Design review of the part built by this model. Coordinates are the model's own, in mm. Coordinates: 2 decimals unless noted, no trailing zeros. Write each loop counter-clockwise with the first axis right and the second up, starting at its lowest first coordinate (ties: lowest second). Pieces come first, ordered by that corner, then holes.
Q1. For L1, parallel to Z at x = -53.73, y = 1.65 (3 decimals); L2, parallel to X at y = 0.75, z = -48.73 (3 decimals); L3, parallel to X at y = 1.7, z = -49, list the stretches that pass through material, from the lowest coordinate up.
Q2. For pin 1 Ø8 at (x, z) = (-26.5, -44) entering from -Y; pin 2 Ø1 at (x, y) = (-42, 1) entering from +Z; pin 3 Ø1 at (y, z) = (1, -48) entering from -X, all flat-tipped, find the tip position at first contact; note any pin that passes through.
Q3. Take a section at A-A, the plane y = 0.75. State how many separate pieces and enclosed holes the cut face has, plus the area to 3 significant figures.
Q4. Take a section at C-C, the plane x = -31.5. Write out the cut boundary in (y, z), plus the area to 3 significant figures.
Q5. Take a section at B-B, the plane z = -7. Write out the cut boundary in (x, y), plus the area to 3 significant figures.
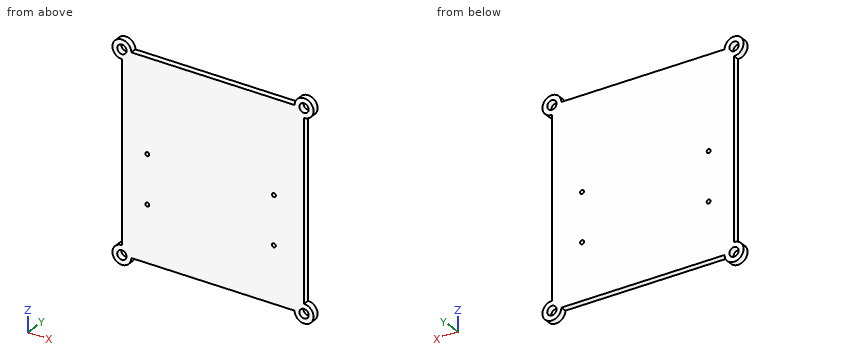
Autodesk Inventor part; units mm, degrees
ref_plane "YZ Plane" through (0, 0, 0) normal (1, 0, 0) x (0, 1, 0)
ref_plane "XZ Plane" through (0, 0, 0) normal (0, 1, 0) x (-1, 0, 0)
ref_plane "XY Plane" through (0, 0, 0) normal (0, 0, 1) x (1, 0, 0)
sketch "Sketch1" plane through (0, 0, 0) normal (0, 1, 0) x (-1, 0, 0)
  line L0 (0, 0) -> (65, 0)
  line L1 (65, 0) -> (65, -70)
  line L2 (65, -70) -> (0, -70)
  line L3 (0, -70) -> (0, 0)
  dimension "d0" = 65
  dimension "d1" = 70
extrude "Extrusion1" add sketch "Sketch1" along normal blind 2
sketch "Sketch2" plane through (0, 2, 0) normal (0, 1, 0) x (1, 0, 0)
  line L0 (0, 70) -> (-65, 70)
  line L1 (-32.5, 69) -> (-10.5, 69)
  line L2 (-32.5, 69) -> (-54.5, 69)
  line L3 (-10.5, 69) -> (-10.5, 55)
  line L4 (-10.5, 55) -> (-54.5, 55)
  line L5 (-54.5, 55) -> (-54.5, 69)
  line L6 (-65, 0) -> (0, 0)
  line L7 (-32.4987, 3) -> (-20.9987, 3)
  line L8 (-32.4987, 3) -> (-43.9987, 3)
  line L9 (-11.55, 31.8) -> (-55, 31.8)
  line L10 (-11.55, 31.8) -> (-11.55, 50)
  line L11 (-55, 31.8) -> (-55, 50)
  line L12 (-55, 50) -> (-11.55, 50)
  line L13 (-20.9987, 3) -> (-20.9987, 19)
  line L14 (-20.9987, 19) -> (-43.9987, 19)
  line L15 (-43.9987, 19) -> (-43.9987, 3)
  line L16 (-20.9987, 19) -> (-20.9987, 16.39)
  line L17 (-20.9987, 19) -> (-20.9987, 16.08)
  line L18 (-55, 50) -> (-53.73, 50)
  circle A0 centre (-53.73, 48.73) radius 0.635
  circle A1 centre (-53.73, 33.07) radius 0.635
  circle A2 centre (-12.82, 48.73) radius 0.635
  circle A3 centre (-12.82, 33.07) radius 0.635
  point P0 (-2, 70)
  point P1 (-63, 70)
  point P2 (-63, 0)
  point P3 (-2, 0)
  dimension "d20" = 18.2
  dimension "d27" = 23
  dimension "d54" = 1.27
  dimension "d56" = 1.27
  dimension "d58" = 1.27
  dimension "d60" = 43.45
  dimension "d63" = 1.27
  dimension "d64" = 1.27
extrude "Extrusion2" cut sketch "Sketch2" against normal blind 2 contours A0 | A1 | A2 | A3
sketch "Sketch4" plane through (0, 2, 0) normal (0, 1, 0) x (1, 0, 0)
  arc A0 (-63, 70) -> (-65, 68) centre (-63, 68) ccw
  line L0 (-63, 68) -> (-61.5, 68) construction
  circle A1 centre (-61.9393, 66.9393) radius 1.5
  arc A2 (0, 68) -> (-2, 70) centre (-2, 68) ccw
  arc A3 (-65, 2) -> (-63, 0) centre (-63, 2) ccw
  arc A4 (-2, 0) -> (0, 2) centre (-2, 2) ccw
  line L1 (-2, 68) -> (-0.5, 68) construction
  circle A5 centre (-3.0607, 66.9393) radius 1.5
  line L2 (-63, 2) -> (-61.5, 2) construction
  circle A6 centre (-61.9393, 3.0607) radius 1.5
  arc A7 (-2, 0) -> (0, 2) centre (-2, 2) ccw
  line L3 (-2, 2) -> (-0.5, 2) construction
  circle A8 centre (-3.0607, 3.0607) radius 1.5
  point P0 (0, 0)
  dimension "d69" = 3
  dimension "d72" = 3
  dimension "d75" = 3
  dimension "d78" = 3
extrude "Extrusion3" cut sketch "Sketch4" against normal blind 2
sketch "Sketch5" plane through (0, 2, 0) normal (0, 1, 0) x (1, 0, 0)
  circle A0 centre (-3.0607, 3.0607) radius 1.5
  circle A1 centre (-3.0607, 66.9393) radius 1.5
  circle A2 centre (-61.9393, 3.0607) radius 1.5
  circle A3 centre (-61.9393, 66.9393) radius 1.5
  circle A4 centre (-12.82, 48.73) radius 0.635
  circle A5 centre (-53.73, 33.07) radius 0.635
  circle A6 centre (-12.82, 33.07) radius 0.635
  circle A7 centre (-53.73, 48.73) radius 0.635
  line L0 (-65, 70) -> (-65, 0)
  line L1 (-65, 0) -> (0, 0)
  line L2 (0, 0) -> (0, 70)
  line L3 (0, 70) -> (-65, 70)
  circle A8 centre (-61.9393, 3.0607) radius 1.5
  circle A9 centre (-3.0607, 66.9393) radius 1.5
  line L4 (-61.9393, 3.0607) -> (-3.0607, 3.0607)
  line L5 (-3.0607, 3.0607) -> (-3.0607, 66.9393)
  line L6 (-3.0607, 66.9393) -> (-61.9393, 66.9393)
  line L7 (-61.9393, 66.9393) -> (-61.9393, 3.0607)
  circle A10 centre (-61.9393, 3.0607) radius 3.0607
  line L8 (-65, 0) -> (0, 0)
  circle A11 centre (-61.9393, 66.9393) radius 1.5
  circle A12 centre (-61.9393, 66.9393) radius 3.0607
  line L9 (0, 70) -> (-65, 70)
  circle A13 centre (-3.0607, 66.9393) radius 1.5
  circle A14 centre (-3.0607, 66.9393) radius 3.0607
  circle A15 centre (-3.0607, 3.0607) radius 1.5
  circle A16 centre (-3.0607, 3.0607) radius 3.0607
  line L10 (0, 0) -> (0, 70)
  line L11 (0, 3.0607) -> (0, 0)
  line L12 (0, 0) -> (-3.0607, 0)
  line L13 (0, 66.9393) -> (0, 70)
  line L14 (0, 70) -> (-3.0607, 70)
  line L15 (-65, 70) -> (-65, 0)
  line L16 (-61.9393, 70) -> (-65, 70)
  line L17 (-65, 70) -> (-65, 66.9393)
  line L18 (-65, 3.0607) -> (-65, 0)
  line L19 (-65, 0) -> (-61.9393, 0)
  point P0 (-3.0607, 0)
extrude "Extrusion4" cut sketch "Sketch5" against normal blind 2 contours L2 L1 A16 | A14 L3 L2 | L1 L0 A10 | A12 L0 L3
sketch "Sketch6" plane through (0, 2, 0) normal (0, 1, 0) x (1, 0, 0)
  arc A0 (0, 66.9393) -> (-3.0607, 70) centre (-3.0607, 66.9393) ccw
  line L0 (-3.0607, 70) -> (-61.9393, 70)
  arc A1 (-61.9393, 70) -> (-65, 66.9393) centre (-61.9393, 66.9393) ccw
  line L1 (-65, 66.9393) -> (-65, 3.0607)
  arc A2 (-65, 3.0607) -> (-61.9393, 0) centre (-61.9393, 3.0607) ccw
  line L2 (-61.9393, 0) -> (-3.0607, 0)
  arc A3 (-3.0607, 0) -> (0, 3.0607) centre (-3.0607, 3.0607) ccw
  line L3 (0, 3.0607) -> (0, 66.9393)
  circle A4 centre (-3.0607, 3.0607) radius 1.5
  circle A5 centre (-3.0607, 66.9393) radius 1.5
  circle A6 centre (-61.9393, 3.0607) radius 1.5
  circle A7 centre (-61.9393, 66.9393) radius 1.5
  circle A8 centre (-12.82, 48.73) radius 0.635
  circle A9 centre (-53.73, 33.07) radius 0.635
  circle A10 centre (-12.82, 33.07) radius 0.635
  circle A11 centre (-53.73, 48.73) radius 0.635
  circle A12 centre (-3.0607, 66.9393) radius 3.0607
  circle A13 centre (-3.0607, 3.0607) radius 1.5
  circle A14 centre (-3.0607, 3.0607) radius 3.0607
  circle A15 centre (-61.9393, 3.0607) radius 1.5
  circle A16 centre (-61.9393, 3.0607) radius 3.0607
  circle A17 centre (-61.9393, 66.9393) radius 1.5
  circle A18 centre (-61.9393, 66.9393) radius 3.0607
  line L4 (-58.8787, 3.0607) -> (-6.1213, 3.0607)
  line L5 (-3.0607, 6.1213) -> (-3.0607, 63.8787)
  line L6 (-6.1213, 66.9393) -> (-58.8787, 66.9393)
  line L7 (-61.9393, 63.8787) -> (-61.9393, 6.1213)
  arc A19 (-65, 3.0607) -> (-61.9393, 0) centre (-61.9393, 3.0607) ccw
  line L8 (-61.9393, 0) -> (-3.0607, 0)
  line L9 (-61.9393, 0) -> (-3.0607, 0)
  line L10 (-65, 3.0607) -> (-65, 66.9393)
  line L11 (-3.0607, 70) -> (-61.9393, 70)
  line L12 (-61.9393, 70) -> (-3.0607, 70)
  arc A20 (0, 66.9393) -> (-3.0607, 70) centre (-3.0607, 66.9393) ccw
  line L13 (0, 3.0607) -> (0, 66.9393)
  line L14 (0, 3.0607) -> (0, 66.9393)
  point P0 (0, 0)
  point P1 (-65, 3.0607)
  point P2 (-3.0607, 0)
extrude "Extrusion5" cut sketch "Sketch6" against normal blind 2 contours L3 A14 L5 A12 | A12 L6 A18 L0 | L2 A16 L4 A14 | A18 L7 A16 L1
properties part number "base" material "Steel, Mild, Welded"
Responses:
1. L1: z = -66.939 to -49.365, -48.095 to -33.705, -32.435 to -3.061
1. L2: x = -61.939 to -54.365, -53.095 to -13.455, -12.185 to -3.061
1. L3: x = -61.94 to -54.3, -53.16 to -13.39, -12.25 to -3.06
2. pin 1: stops at y = 0
2. pin 2: stops at z = -3.06
2. pin 3: stops at x = -61.94
3. separate pieces: 1
3. enclosed holes: 8
3. area: 3,820 mm2
4. outline: (0, -66.94) - (2, -66.94) - (2, -3.06) - (0, -3.06) - close
4. area: 128 mm2
5. outline: (-61.94, 0) - (-3.06, 0) - (-3.06, 2) - (-61.94, 2) - close
5. area: 118 mm2
